Part print with two shaded views. Sizes in mm from the minimum x, y, z corner. Coordinates: 2 decimals unless noted, no trailing zeros. Loops run counter-clockwise (first coordinate to the right, second up) from the corner with the lowest first, then second, coordinate; pieces in that order, holes last. Notation, with made-up numbers: M 31.25,-24.5 L 75.25,-24.5 A26 ccw 75.25,-9.5 Z; hole C 67.5,74.5 d9. An arc over 180 degrees is marked long. Write item = value, one per line. Start each with the question number.
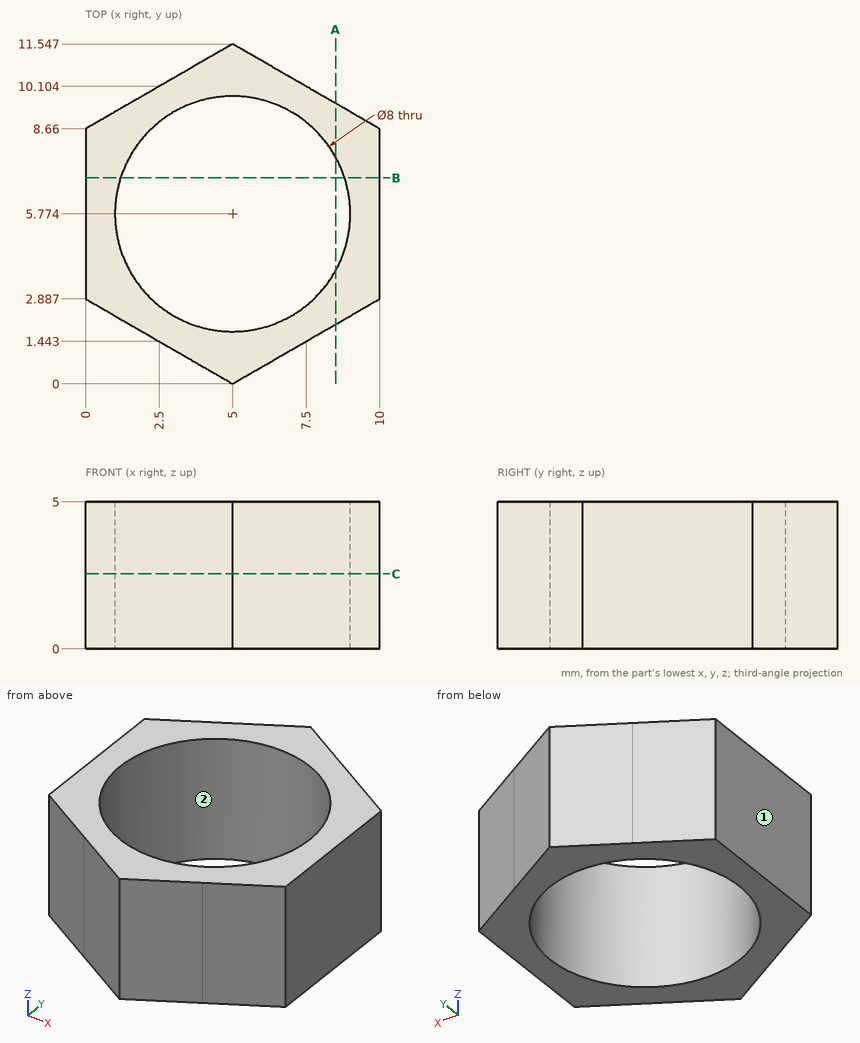
Item 1: Pin check, flat tip, straight feed: pin 1 Ø6 at (x, y) = (2, 9) entering from -Z. Stop position of the tip, or through.
Item 2: Probe L1, parallel to Y at x = 4, z = 3 (1 decimal); L2, parallel to X at y = 3.25, z = 4.45 (1 decimal); L3, parallel to X at y = 5.25, z = 3.6 (1 decimal). List the from-to ranges inside material, lowest first.
Item 3: Cut at C-C (z = 2.55). Give the cut face in (x, y).
Item 4: Cut at A-A (x = 8.5). Give the cut face in (y, z).
Item 5: Pull direction Y, two halves, no side cores. Call the marked faces 1 and 2: +Y half, -Y half, draft (parallel to the pull), parting line (faces both ways), or undercut.
Item 6: Cut at B-B (y = 7). Give the cut face in (x, z).
Reported:
q1.pin_1 = 0
q2.L1 = 0.6 to 1.9, 9.6 to 11
q2.L2 = 0 to 1.9, 8.1 to 10
q2.L3 = 0 to 1, 9 to 10
q3.outline = M 0,2.89 L 5,0 L 10,2.89 L 10,8.66 L 5,11.55 L 0,8.66 Z; hole C 5,5.77 d8
q4.outline = M 2.02,0 L 3.84,0 L 3.84,5 L 2.02,5 Z; M 7.71,0 L 9.53,0 L 9.53,5 L 7.71,5 Z
q5.face_1 = draft
q5.face_2 = undercut
q6.outline = M 0,0 L 1.19,0 L 1.19,5 L 0,5 Z; M 8.81,0 L 10,0 L 10,5 L 8.81,5 Z
